Build history of the part. All positions in model axes, mm. Coordinates: 2 decimals unless noted, no trailing zeros. Order: outer loops, then holes, each group sorted by start corner. A loop starts at its lowest first (then second) coordinate and runs counter-clockwise, first axis right, second up. Notation, with made-up numbers: (5, 80) -> (60, 80) arc R27 cw to (60, 106) -> close; hole circle Ø2 at (83.5, 45.25). An arc over 180 degrees is marked (long way). Write each question's results on one line, items separated by ' | '.
from build123d import *

# Parameters (mm, degrees)
SKETCH2_W           = 71.882
SKETCH2_H           = 76.2
BOSS_EXTRUDE2_DEPTH = 5.2578
CAVITY1_START       = 9.525
CAVITY1_OUTLINE_R   = 1.7526
CAVITY1_DEPTH       = 5.2578
FILLET3_R           = 12.7
FILLET4_R           = 12.7
FILLET5_R           = 12.7
FILLET6_R           = 12.7


# Read off the part's stored shape, not the designer's step: Cavity1
with BuildPart() as part:
    # Sketch2 → Boss-Extrude2 (new body)
    with BuildSketch(Plane(origin=(0, 9.525, 0), x_dir=(1, 0, 0), z_dir=(0, 1, 0))):
        with Locations((4.191, 35.4711)):
            Rectangle(SKETCH2_W, SKETCH2_H)
    extrude(amount=BOSS_EXTRUDE2_DEPTH)

    # Cavity1 outline → Cavity1 (cut)
    with BuildSketch(Plane(origin=(0, 0, 0), x_dir=(1, 0, 0), z_dir=(0, 1, 0)).offset(CAVITY1_START)):
        with Locations((25.576048817, 12.7)):
            Circle(CAVITY1_OUTLINE_R)
        with Locations((-17.177400647, 12.7)):
            Circle(CAVITY1_OUTLINE_R)
    extrude(amount=CAVITY1_DEPTH, mode=Mode.SUBTRACT)

    # Fillet3
    fillet3_edges = [part.edges().sort_by_distance(p)[0] for p in [
        (40.132, 12.1539, 2.6289),
    ]]
    fillet(fillet3_edges, radius=FILLET3_R)

    # Fillet4
    fillet4_edges = [part.edges().sort_by_distance(p)[0] for p in [
        (-31.75, 12.1539, 2.6289),
    ]]
    fillet(fillet4_edges, radius=FILLET4_R)

    # Fillet5
    fillet5_edges = [part.edges().sort_by_distance(p)[0] for p in [
        (40.132, 12.1539, -73.5711),
    ]]
    fillet(fillet5_edges, radius=FILLET5_R)

    # Fillet6
    fillet6_edges = [part.edges().sort_by_distance(p)[0] for p in [
        (-31.75, 12.1539, -73.5711),
    ]]
    fillet(fillet6_edges, radius=FILLET6_R)


solid = part.part
Item 1: Drill centre lines: line 1 (X direction, y = 11.5, z = -12.7); line 2 (Z direction, x = -16, y = 13.1); line 3 (X direction, y = 11.6, z = -63). Where is each one in solid material? Low to high. Write a range as from..to.
Answer:
line 1: x = -31.75..-18.93, -15.42..23.82, 27.33..40.13 | line 2: z = -73.57..-14, -11.4..2.63 | line 3: x = -31.57..39.95
Item 2: Slice it at D-D, the plane z = -4. List the corners of the cut face in (x, y) (3 decimals), and give its area (3 significant figures).
Answer:
outline: (-30.205, 9.525) -> (38.587, 9.525) -> (38.587, 14.783) -> (-30.205, 14.783) -> close | area: 362 mm^2
Item 3: Slice it at A-A, the plane z = -12.7. List the corners of the cut face in (x, y) (3 decimals), and give its area (3 significant figures).
Answer:
outline: (-31.75, 9.525) -> (-18.93, 9.525) -> (-18.93, 14.783) -> (-31.75, 14.783) -> close; (-15.425, 9.525) -> (23.823, 9.525) -> (23.823, 14.783) -> (-15.425, 14.783) -> close; (27.329, 9.525) -> (40.132, 9.525) -> (40.132, 14.783) -> (27.329, 14.783) -> close | area: 341 mm^2
Item 4: Slice it at B-B, the plane y = 12.8. List the corners of the cut face in (x, z), and give its area (3 significant figures).
Answer:
outline: (-31.75, -60.87) arc R12.7 ccw to (-19.05, -73.57) -> (27.43, -73.57) arc R12.7 ccw to (40.13, -60.87) -> (40.13, -10.07) arc R12.7 ccw to (27.43, 2.63) -> (-19.05, 2.63) arc R12.7 ccw to (-31.75, -10.07) -> close; hole circle Ø3.51 at (-17.18, -12.7); hole circle Ø3.51 at (25.58, -12.7) | area: 5,320 mm^2
Item 5: Slice it at C-C, the plane x = 34.5. List the corners of the cut face in (y, z) (3 decimals).
Answer:
outline: (9.525, -71.423) -> (14.783, -71.423) -> (14.783, 0.48) -> (9.525, 0.48) -> close
Item 6: Pin check, flat tips, straight feed: pin 1 (2 mm diameter, centred on x = -17.18, z = -12.7, fed in from +Y); pin 2 (3 mm diameter, centred on y = 13.5, z = -6.5, fed in from +X). Stop position of each tip, or through.
Answer:
pin 1: passes through | pin 2: stops at x = 39.96
Item 7: Pull direction X, two halves, no side cores. Call faces 1 (the flat face through (4, 12, 2.629)), 2 (the cylindrical face through (36.31, 12.19, -0.99)), 3 (the cylindrical face through (24.19, 12.12, -11.63)): released by +X, released by -X, zero draft, split by the parting line, or undercut.
Answer:
face 1: zero draft | face 2: released by +X | face 3: undercut
